```python
from build123d import *

# Parameters (mm, degrees)
SKETCH7_R          = 13
SKETCH7_R_2        = 8
CUT_EXTRUDE3_DEPTH = 3
SKETCH6_R          = 1.7
CUT_EXTRUDE2_DEPTH = 8


with BuildPart() as part:
    # Sketch1 → Revolve1 (revolve)
    with BuildSketch(Plane.XY):
        Polygon((-0.2, 0), (-0.2, 8), (-1.6, 8.841204867), (-1.6, 11), (-3.25, 11.991420021), (-3.25, 20.948493917), (-5, 22), (-5, 29), (-11, 32.605163714), (-11, 116), (-13, 116), (-13, 0), align=None)
    revolve(axis=Axis((0, 0, 0), (0, 1, 0)))

    # Sketch7 → Cut-Extrude3 (cut)
    with BuildSketch(Plane.XZ):
        Circle(SKETCH7_R)
        Circle(SKETCH7_R_2, mode=Mode.SUBTRACT)
    extrude(amount=-CUT_EXTRUDE3_DEPTH, mode=Mode.SUBTRACT)

    # Sketch6 → Cut-Extrude2 (cut)
    with BuildSketch(Plane.XY.offset(13)):
        with Locations((0, 7)):
            Circle(SKETCH6_R)
    extrude(amount=-CUT_EXTRUDE2_DEPTH, mode=Mode.SUBTRACT)


solid = part.part
```
The listing builds one solid part. Answer for the finished solid, in the listing's coordinates (mm). A direction names the side the tool comes from. Coordinates: 2 decimals unless noted, no trailing zeros. Write each loop counter-clockwise with the first axis right and the second up, starting at its lowest first coordinate (ties: lowest second). Pieces come first, ordered by that corner, then holes. Notation, with made-up numbers: (-14.5, 46.5) - (32.5, 46.5) arc R36 ccw to (32.5, 84.5) - close; hole circle Ø1 at (-8, 41). An arc over 180 degrees is marked (long way). Return JSON: item names as keys, results as strings. Group by question number.
1. A cutting plane is placed at A-A, the plane y = 10. Determine the outline of the cut face in (x, z), plus the area to 3 significant figures.
2. Straight lines are drawn through the part: L1, parallel to X at y = 41, z = 0.25; L2, parallel to Z at x = 0, y = 25.5; L3, parallel to Z at x = -10.25, y = 14.5. For each, find the intervals that lie inside material, in ascending order.
3. Determine the mould class of faces 4 (the cylindrical face through (-0.37, 5.34, 9.06)), 5 (the flat face through (-11, 116, 3)), 6 (the flat face through (0, 7, 5)), 7 (the cylindrical face through (2.38, 74.89, -10.74)) for opening direction Y: released by +Y, released by -Y, zero draft, split by the parting line, or undercut.
4. Given pin 1 (3 mm diameter, centred on x = -8, y = 50, fed in from +Z); pin 2 (5 mm diameter, centred on x = 9, z = 1, fed in from +Y); pin 3 (4 mm diameter, centred on x = 0, z = 0, fed in from +Y); pin 4 (2 mm diameter, centred on y = 39.5, z = 1.5, fed in from +X), each flat-ended and moving along its own axis, determine where each tip first touches the part or whether it passes through.
5. Which of the six approach directions +Z, -Z, +X, -X, +Y, -Y give full straight-line access (tool end or side, diameter ignored) to faces 1 (the cylindrical face through (10.316, 58.709, -7.91)), 2 (the cylindrical face through (1.27, 9.94, -0.97)), 3 (the cylindrical face through (-1.73, 1.48, -7.81))?
6. A cutting plane is placed at B-B, the plane y = 97. Determine the outline of the cut face in (x, z), plus the area to 3 significant figures.
Ans:
{
 "1": {"outline": "circle Ø26 at (0, 0); hole circle Ø3.2 at (0, 0)", "area": "523 mm²"},
 "2": {"L1": "-13 to -11, 11 to 13", "L2": "-13 to -5, 5 to 13", "L3": "-8 to 8"},
 "3": {"face 4": "undercut", "face 5": "released by +Y", "face 6": "undercut", "face 7": "zero draft"},
 "4": {"pin 1": "z = 11.26", "pin 2": "y = 116", "pin 3": "y = 11.24", "pin 4": "x = 12.99"},
 "5": {"face 1": "+Y, -Y", "face 2": "+Y", "face 3": "-Y"},
 "6": {"outline": "circle Ø26 at (0, 0); hole circle Ø22 at (0, 0)", "area": "151 mm²"}
}
